from build123d import *

# Parameters (mm, degrees)
SKETCH_3_R          = 2.15
CUT_EXTRUDE_2_DEPTH = 10


with BuildPart() as part:
    # 草图1 → 旋转1 (revolve)
    with BuildSketch(Plane.XY, mode=Mode.PRIVATE) as revolve_1_sk:
        Polygon((44.5, 0), (58, 0), (61, 0), (61, 9.1), (58, 9.1), (58, 6.1), (44.5, 6.1), align=None)
    revolve(revolve_1_sk.sketch.rotate(Axis((0, 0, 0), (0, 1, 0)), 90), axis=Axis((0, 0, 0), (0, 1, 0)))

    # 草图3 → 切除-拉伸2 (cut)
    with BuildSketch(Plane(origin=(0, 6.1, 0), x_dir=(1, 0, 0), z_dir=(0, 1, 0))):
        with Locations(Location((-50.45, 0, 0), (0, 0, 270))):
            Circle(SKETCH_3_R)
        with Locations(Location((-25.225, 43.690981621, 0), (0, 0, 270))):
            Circle(SKETCH_3_R)
        with Locations(Location((25.225, 43.690981621, 0), (0, 0, 270))):
            Circle(SKETCH_3_R)
        with Locations(Location((50.45, 0, 0), (0, 0, 270))):
            Circle(SKETCH_3_R)
        with Locations(Location((25.225, -43.690981621, 0), (0, 0, 270))):
            Circle(SKETCH_3_R)
        with Locations(Location((-25.225, -43.690981621, 0), (0, 0, 270))):
            Circle(SKETCH_3_R)
    extrude(amount=-CUT_EXTRUDE_2_DEPTH, mode=Mode.SUBTRACT)


solid = part.part
The model under review builds one solid part; all positions refer to its coordinate system, in mm. A direction names the side the tool comes from. Give positions to 0.01 mm unless a question says otherwise; leave off trailing zeros. Order: outer loops, then holes, each group sorted by start corner. A loop starts at its lowest first (then second) coordinate and runs counter-clockwise, first axis right, second up. Notation, with made-up numbers: M 33,7 L 64,7 A28 ccw 64,33 Z; hole C -20.5,48 d10. An arc over 180 degrees is marked long. Answer in a Markdown table with one row per item. Add a question column.
1. Add section D-D on x = -39. State the section outline as (y, z) points.
2. To check wall thickness, follow line 1 along X through (y, z) = (1.5, 0); line 2 along Z through (x, y) = (26, 4); line 3 along Y through (x, z) = (-9.5, -48.5). State the ranges of each line that lie inside material, in increasing order.
3. For pin 1 Ø1 at (y, z) = (2.5, -13) entering from +X; pin 2 Ø8 at (x, z) = (16, 43) entering from -Y; pin 3 Ø7 at (x, z) = (-50.45, 0) entering from +Y; pin 4 Ø3.5 at (x, z) = (50.45, 0) entering from +Y, all flat-tipped, find the tip position at first contact; note any pin that passes through.
4. Add section B-B on x = 0. State the section outline as (y, z) points, plus the area to 3 significant figures.
5. Mouldability with a two-part tool opening along X and no side actions: class faces 1 (the cylindrical face through (59.55, 4.61, 13.22)), 2 (the flat face through (54, 9.1, -22)), 3 (the cylindrical face through (-30.075, 3.007, 32.798)) as released by +X, released by -X, zero draft, split by the parting line, or undercut.
6. Add section C-C on y = 2. State the section outline as (x, z) points (3 decimals), plus the area to 3 significant figures.
7. Add section A-A on z = 0. State the section outline as (x, y) points.
8. Machinability: for faces 4 (the cylindrical face through (-52.55, 3.09, -0.47)), 5 (the flat face through (43, 6.1, -13)), which of the approach directions +Z, -Z, +X, -X, +Y, -Y give a long, thin tool a straight path to every point of the face, cutting with its end or side? Answer none if there is none.
The answers:
| question | item | result |
|---|---|---|
| 1 | outline | M 0,-46.9 L 9.1,-46.9 L 9.1,-42.93 L 6.1,-42.93 L 6.1,-21.43 L 0,-21.43 Z; M 0,21.43 L 6.1,21.43 L 6.1,42.93 L 9.1,42.93 L 9.1,46.9 L 0,46.9 Z |
| 2 | line 1 | -61 to -52.6, -48.3 to -44.5, 44.5 to 48.3, 52.6 to 61 |
| 2 | line 2 | -55.18 to -45.7, -41.69 to -36.11, 36.11 to 41.69, 45.7 to 55.18 |
| 2 | line 3 | 0 to 6.1 |
| 3 | pin 1 | x = 59.71 |
| 3 | pin 2 | y = 0 |
| 3 | pin 3 | y = 6.1 |
| 3 | pin 4 | through |
| 4 | outline | M 0,-61 L 9.1,-61 L 9.1,-58 L 6.1,-58 L 6.1,-44.5 L 0,-44.5 Z; M 0,44.5 L 6.1,44.5 L 6.1,58 L 9.1,58 L 9.1,61 L 0,61 Z |
| 4 | area | 219 mm2 |
| 5 | face 1 | split by the parting line |
| 5 | face 2 | zero draft |
| 5 | face 3 | undercut |
| 6 | outline | C 0,0 d122; hole C -50.45,0 d4.3; hole C 0,0 d89; hole C -25.225,-43.691 d4.3; hole C -25.225,43.691 d4.3; hole C 25.225,-43.691 d4.3; hole C 25.225,43.691 d4.3; hole C 50.45,0 d4.3 |
| 6 | area | 5,380 mm2 |
| 7 | outline | M -61,0 L -52.6,0 L -52.6,6.1 L -58,6.1 L -58,9.1 L -61,9.1 Z; M -48.3,0 L -44.5,0 L -44.5,6.1 L -48.3,6.1 Z; M 44.5,0 L 48.3,0 L 48.3,6.1 L 44.5,6.1 Z; M 52.6,0 L 61,0 L 61,9.1 L 58,9.1 L 58,6.1 L 52.6,6.1 Z |
| 8 | face 4 | +Y, -Y |
| 8 | face 5 | +Y |
